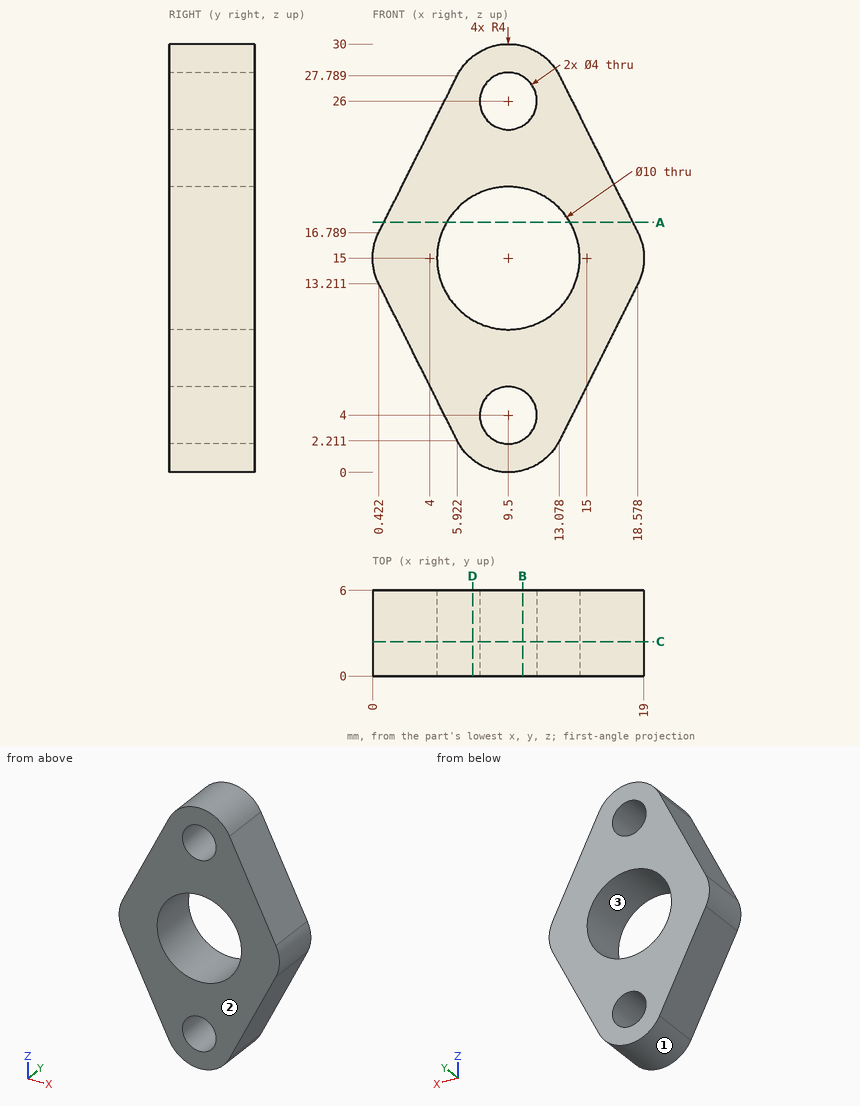
Check sheet for the drawn part. Datum: minimum x, y, z corner. Units: mm. Give positions to 0.01 mm unless a question says otherwise; leave off trailing zeros. Write each loop counter-clockwise with the first axis right and the second up, starting at its lowest first coordinate (ties: lowest second). Pieces come first, ordered by that corner, then holes. Notation, with made-up numbers: (84.5, 23) -> (89.5, 23) arc R30 ccw to (89.5, 53) -> close; hole circle Ø4 at (84.5, 41). An arc over 180 degrees is marked (long way). Use one line per item in the form item = value. Start each with the question number.
1. Thickness scan on line 1 along X through (y, z) = (3.4, 15); line 2 along Z through (x, y) = (8.5, 3.5); line 3 along Z through (x, y) = (9.25, 2.3) (1 decimal). Record the ranges inside material, lowest first. Write a range as from..to.
2. Section check D-D (x = 7). Record the cut outline in (y, z).
3. Section check C-C (y = 2.4). Record the cut outline in (x, z).
4. Go/stop test with flat-tipped pins: P1, Ø2, axis at x = 5, y = 1, coming from the +Z side (1 decimal); P2, Ø3, axis at x = 16.5, y = 1.5, coming from the +Z side (1 decimal); P3, Ø1, axis at x = 12, z = 12.5, coming from the +Y side; P4, Ø1.5, axis at y = 0.5, z = 16.5, coming from the +X side. Record where each tip stops, or that it passes through.
5. Section check A-A (z = 17.5). Record the cut outline in (x, y), and give its area (3 significant figures).
6. Section check B-B (x = 10.5). Record the cut outline in (y, z).
7. Mould release check, pull along X, two halves, no side actions. Record for the marked faces 1, 2 and 3: pulls with the +X half, pulls with the -X half, needs draft (parallel to the pull), parting line crosses it, or undercut.
Conclusion:
q1.line_1 = 0..4.5, 14.5..19
q1.line_2 = 0.13..2.27, 5.73..10.1, 19.9..24.27, 27.73..29.87
q1.line_3 = 0..2, 6..10, 20..24, 28..30
q2.outline = (0, 0.88) -> (6, 0.88) -> (6, 10.67) -> (0, 10.67) -> close; (0, 19.33) -> (6, 19.33) -> (6, 29.12) -> (0, 29.12) -> close
q3.outline = (0.42, 13.21) -> (5.92, 2.21) arc R4 ccw to (13.08, 2.21) -> (18.58, 13.21) arc R4 ccw to (18.58, 16.79) -> (13.08, 27.79) arc R4 ccw to (5.92, 27.79) -> (0.42, 16.79) arc R4 ccw to start; hole circle Ø10 at (9.5, 15); hole circle Ø4 at (9.5, 4); hole circle Ø4 at (9.5, 26)
q4.P1 = 27.9
q4.P2 = 23.9
q4.P3 = through
q4.P4 = 18.93
q5.outline = (0.78, 0) -> (5.17, 0) -> (5.17, 6) -> (0.78, 6) -> close; (13.83, 0) -> (18.22, 0) -> (18.22, 6) -> (13.83, 6) -> close
q5.area = 52.7 mm²
q6.outline = (0, 0.13) -> (6, 0.13) -> (6, 2.27) -> (0, 2.27) -> close; (0, 5.73) -> (6, 5.73) -> (6, 10.1) -> (0, 10.1) -> close; (0, 19.9) -> (6, 19.9) -> (6, 24.27) -> (0, 24.27) -> close; (0, 27.73) -> (6, 27.73) -> (6, 29.87) -> (0, 29.87) -> close
q7.face_1 = parting line crosses it
q7.face_2 = needs draft
q7.face_3 = undercut
